For this review, take the finished solid that the model builds, in its own axes (mm). A direction names the side the tool comes from. Give positions to 0.01 mm unless a question says otherwise; leave off trailing zeros. Order: outer loops, then holes, each group sorted by start corner. A loop starts at its lowest first (then second) coordinate and runs counter-clockwise, first axis right, second up. Notation, with made-up numbers: M 17.25,58.25 L 39.25,58.25 A12 cw 39.25,64.25 Z; hole C -20.5,88 d10. An arc over 180 degrees is marked long. Answer as CSV lines item,"result". Start each with the question number.
1. Machinability: for faces 4 (the flat face through (-0.8, 0.1, 115)), 5 (the flat face through (-4, -12.1, 2)), which of the approach directions +Z, -Z, +X, -X, +Y, -Y give a long, thin tool a straight path to every point of the face, cutting with its end or side? Answer none if there is none.
2. We need section C-C, the plane y = 1.5. Give the boundary of the cut face in (x, z), and give its area (3 significant figures).
3. Mouldability with a two-part tool opening along X and no side actions: class faces 1 (the flat face through (0, 0, 2)), 2 (the flat face through (-4, 12.1, 2)), 3 (the flat face through (-4, -13.1, 2)) as pulls with the +X half, pulls with the -X half, needs draft (parallel to the pull), parting line crosses it, or undercut.
4. For line 1 along Y through (x, z) = (-1.75, 8); line 2 along X through (y, z) = (9.25, -55.5); line 3 along X through (y, z) = (-11.5, 39), list the stretches that pass through material, from the lowest coordinate up.
5. We need section B-B, the plane z = 1.5. Give the boundary of the cut face in (x, y).
6. We need section A-A, the plane x = -5. Give the boundary of the cut face in (y, z), and give its area (3 significant figures).
7. Clearance check with flat-ended pins moving along their axes: P1, Ø1, axis at x = -2.5, y = -3, coming from the +Z side; P2, Ø1.1, axis at x = -8, z = -5, coming from the +Y side; P3, Ø0.5, axis at x = -8, z = -12, coming from the -Y side. State where each tip first meets the part, or that it passes through.
from build123d import *

# Parameters (mm, degrees)
SM_BASE_FLANGE_1_DEPTH = 115


# Sheet-metal steps are written as plain solids
with BuildPart() as part:
    # Sketch 1 → Базовая кромка1 (new, symmetric)
    with BuildSketch(Plane.XY):
        with BuildLine():
            Line((-8.7, 11.1), (-8.7, 11.9))
            ThreePointArc((-8.7, 11.9), (-8.348528137, 12.748528137), (-7.5, 13.1))
            Line((-7.5, 13.1), (-1.2, 13.1))
            ThreePointArc((-1.2, 13.1), (-0.351471863, 12.748528137), (0, 11.9))
            Line((0, 11.9), (0, -11.9))
            ThreePointArc((0, -11.9), (-0.351471863, -12.748528137), (-1.2, -13.1))
            Line((-1.2, -13.1), (-7.5, -13.1))
            ThreePointArc((-7.5, -13.1), (-8.348528137, -12.748528137), (-8.7, -11.9))
            Line((-8.7, -11.9), (-8.7, -11.1))
            Line((-8.7, -11.1), (-7.7, -11.1))
            Line((-7.7, -11.1), (-7.7, -11.9))
            ThreePointArc((-7.7, -11.9), (-7.641421356, -12.041421356), (-7.5, -12.1))
            Line((-7.5, -12.1), (-1.2, -12.1))
            ThreePointArc((-1.2, -12.1), (-1.058578644, -12.041421356), (-1, -11.9))
            Line((-1, -11.9), (-1, 11.9))
            ThreePointArc((-1, 11.9), (-1.058578644, 12.041421356), (-1.2, 12.1))
            Line((-1.2, 12.1), (-7.5, 12.1))
            ThreePointArc((-7.5, 12.1), (-7.641421356, 12.041421356), (-7.7, 11.9))
            Line((-7.7, 11.9), (-7.7, 11.1))
            Line((-7.7, 11.1), (-8.7, 11.1))
        make_face()
    extrude(amount=SM_BASE_FLANGE_1_DEPTH, both=True)


solid = part.part
Result set:
1,face 4,"+Z, +X, -X, +Y, -Y"
1,face 5,"+Z, -Z"
2,outline,"M -1,-115 L 0,-115 L 0,115 L -1,115 Z"
2,area,"230 mm2"
3,face 1,"pulls with the +X half"
3,face 2,"undercut"
3,face 3,"needs draft"
4,line 1,"-13.1 to -12.1, 12.1 to 13.1"
4,line 2,"-1 to 0"
4,line 3,"-8.7 to -7.7, -1 to 0"
5,outline,"M -8.7,-11.9 A1.2 ccw -7.5,-13.1 L -1.2,-13.1 A1.2 ccw 0,-11.9 L 0,11.9 A1.2 ccw -1.2,13.1 L -7.5,13.1 A1.2 ccw -8.7,11.9 L -8.7,11.1 L -7.7,11.1 L -7.7,11.9 A0.2 cw -7.5,12.1 L -1.2,12.1 A0.2 cw -1,11.9 L -1,-11.9 A0.2 cw -1.2,-12.1 L -7.5,-12.1 A0.2 cw -7.7,-11.9 L -7.7,-11.1 L -8.7,-11.1 Z"
6,outline,"M -13.1,-115 L -12.1,-115 L -12.1,115 L -13.1,115 Z; M 12.1,-115 L 13.1,-115 L 13.1,115 L 12.1,115 Z"
6,area,"460 mm2"
7,P1,"through"
7,P2,"y = 13.1"
7,P3,"y = -13.07"
